Part model, mm, in its own coordinate system. Face numbers are marked on the shaded views. Round coordinates to 2 decimals unless told otherwise and drop trailing zeros. Loops run counter-clockwise (first coordinate to the right, second up) from the corner with the lowest first, then second, coordinate; pieces in that order, holes last.
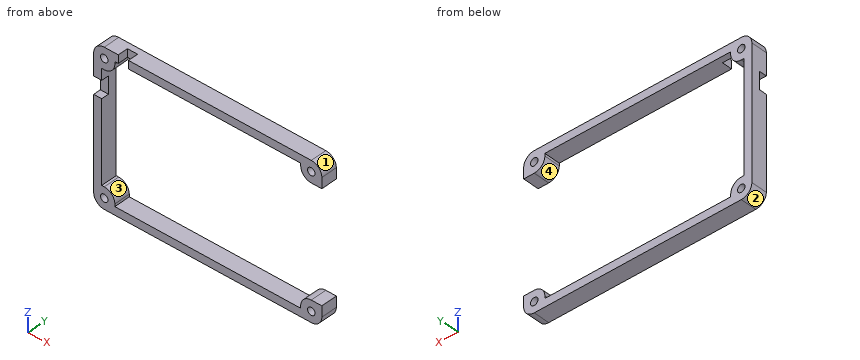
from build123d import *

# Parameters (mm, degrees)
BOSS_EXTRUDE3_DEPTH = 6.35
SKETCH5_W           = 6.8
SKETCH5_H           = 5.9
CUT_EXTRUDE3_DEPTH  = 3.175
SKETCH7_R           = 1.475
SKETCH7_R_2         = 1.4732
CUT_EXTRUDE5_DEPTH  = 6.35
SKETCH8_W           = 3.175
SKETCH8_H           = 43.3
CUT_EXTRUDE6_DEPTH  = 10
SKETCH9_W           = 4
SKETCH9_H           = 4
CUT_EXTRUDE8_DEPTH  = 4


with BuildPart() as part:
    # Sketch2 → Boss-Extrude3 (new body)
    with BuildSketch(Plane(origin=(0, 0, 0), x_dir=(1, 0, 0), z_dir=(0, 1, 0))):
        with BuildLine():
            Line((-45, 25.825), (-45, -25.825))
            ThreePointArc((-45, -25.825), (-43.777170811, -28.777170811), (-40.825, -30))
            Line((-40.825, -30), (40.825, -30))
            ThreePointArc((40.825, -30), (43.777170811, -28.777170811), (45, -25.825))
            Line((45, -25.825), (45, 25.825))
            ThreePointArc((45, 25.825), (43.777170811, 28.777170811), (40.825, 30))
            Line((40.825, 30), (-40.825, 30))
            ThreePointArc((-40.825, 30), (-43.777170811, 28.777170811), (-45, 25.825))
        make_face()
        with BuildLine():
            Line((40.825, 21.65), (41.825, 21.65))
            Line((41.825, 21.65), (41.825, -21.65))
            Line((41.825, -21.65), (40.825, -21.65))
            ThreePointArc((40.825, -21.65), (37.872829189, -22.872829189), (36.65, -25.825))
            Line((36.65, -25.825), (36.65, -26.825))
            Line((36.65, -26.825), (-36.65, -26.825))
            Line((-36.65, -26.825), (-36.65, -25.825))
            ThreePointArc((-36.65, -25.825), (-37.872829189, -22.872829189), (-40.825, -21.65))
            Line((-40.825, -21.65), (-41.825, -21.65))
            Line((-41.825, -21.65), (-41.825, 21.65))
            Line((-41.825, 21.65), (-40.825, 21.65))
            ThreePointArc((-40.825, 21.65), (-37.872829189, 22.872829189), (-36.65, 25.825))
            Line((-36.65, 25.825), (-36.65, 26.825))
            Line((-36.65, 26.825), (36.65, 26.825))
            Line((36.65, 26.825), (36.65, 25.825))
            ThreePointArc((36.65, 25.825), (37.872829189, 22.872829189), (40.825, 21.65))
        make_face(mode=Mode.SUBTRACT)
    extrude(amount=BOSS_EXTRUDE3_DEPTH)

    # Sketch5 → Cut-Extrude3 (cut)
    with BuildSketch(Plane.ZY.offset(45)):
        with Locations((13.825, 0)):
            Rectangle(SKETCH5_W, SKETCH5_H)
    extrude(amount=-CUT_EXTRUDE3_DEPTH, mode=Mode.SUBTRACT)

    # Sketch7 → Cut-Extrude5 (cut)
    with BuildSketch(Plane.XZ):
        with Locations(Location((-40.825, -25.825, 0), (0, 0, 270))):
            Circle(SKETCH7_R)
        with Locations(Location((-40.825, 25.81356336, 0), (0, 0, 270))):
            Circle(SKETCH7_R_2)
        with Locations(Location((40.825, 25.825, 0), (0, 0, 270))):
            Circle(SKETCH7_R_2)
        with Locations(Location((40.825, -25.81487963, 0), (0, 0, 270))):
            Circle(SKETCH7_R_2)
    extrude(amount=-CUT_EXTRUDE5_DEPTH, mode=Mode.SUBTRACT)

    # Sketch8 → Cut-Extrude6 (cut)
    with BuildSketch(Plane(origin=(0, 6.35, 0), x_dir=(1, 0, 0), z_dir=(0, 1, 0))):
        with Locations((43.4125, 0)):
            Rectangle(SKETCH8_W, SKETCH8_H)
    extrude(amount=-CUT_EXTRUDE6_DEPTH, mode=Mode.SUBTRACT)

    # Sketch9 → Cut-Extrude8 (cut)
    with BuildSketch(Plane.XY.offset(30)):
        with Locations((-33.2866, 2)):
            Rectangle(SKETCH9_W, SKETCH9_H)
    extrude(amount=-CUT_EXTRUDE8_DEPTH, mode=Mode.SUBTRACT)


solid = part.part
1) Slice it at A-A, the plane x = -33. Give the cut face in (y, z) (3 decimals), then the cut area to 3 significant figures.
Values:
outline: (0, -30) - (6.35, -30) - (6.35, -26.825) - (0, -26.825) - close; (4, 26.825) - (6.35, 26.825) - (6.35, 30) - (4, 30) - close
area: 27.6 mm2
2) Mould opens along Z. For the marked faces 1, 2, 3 and 4 say: released by +Z, released by -Z, zero draft, split by the parting line, or undercut.
Values:
face 1: released by +Z
face 2: released by -Z
face 3: undercut
face 4: undercut
3) Slice it at D-D, the plane z = -1. Give the cut face in (x, y) (3 decimals), then the cut area to 3 significant figures.
Values:
outline: (-45, 0) - (-41.825, 0) - (-41.825, 6.35) - (-45, 6.35) - close
area: 20.2 mm2
4) Slice it at B-B, the plane y = 1. Give the number of separate pieces and of enclosed holes in the cut face, then the cut area to 3 significant figures.
Values:
separate pieces: 3
enclosed holes: 4
area: 790 mm2
5) Slice it at C-C, the plane z = 23. Give the cut face in (x, y), then the cut area to 3 significant figures.
Values:
outline: (-45, 0) - (-37.75, 0) - (-37.75, 6.35) - (-45, 6.35) - close; (37.75, 0) - (45, 0) - (45, 6.35) - (37.75, 6.35) - close
area: 92.1 mm2
6) Wall check: line 1 along Z through (x, y) = (-29.5, 5.25) (3 decimals); line 2 along Z through (x, y) = (-40, 4.75); line 3 along X through (y, z) = (1, -10.5) (3 decimals). Give the ranges that are in metal, low to high.
Values:
line 1: z = -30 to -26.825, 26.825 to 30
line 2: z = -30 to -27.05, -24.6 to -21.73, 21.73 to 24.59, 27.03 to 30
line 3: x = -45 to -41.825
7) Drop flat-ended pins along their axis: pin 1 Ø0.5 at (y, z) = (4, 26.5) entering from -X; pin 2 Ø3.5 at (y, z) = (1.5, 28) entering from +X; pin 3 Ø3.5 at (y, z) = (1.5, 28.5) entering from -X; pin 4 Ø1.1 at (x, y) = (-41.5, 2) entering from -Z. Give the stop position or say it passes through.
Values:
pin 1: stops at x = -44.98
pin 2: stops at x = 44.98
pin 3: stops at x = -44.9
pin 4: stops at z = -30
